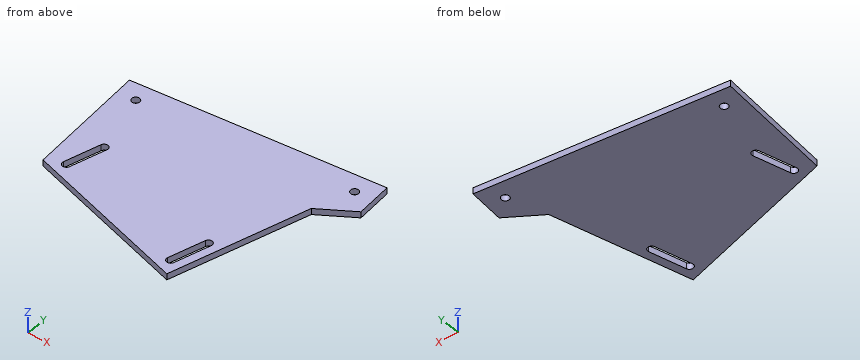
```python
from build123d import *

# Parameters (mm, degrees)
SKETCH2_R           = 4.1021
BOSS_EXTRUDE2_DEPTH = 6.35


with BuildPart() as part:
    # Sketch2 → Boss-Extrude2 (new body)
    with BuildSketch(Plane.XY):
        Polygon((416.876840794, 161.047876949), (163.843387479, 138.910318291), (174.883865248, 12.717079939), (347.922940958, -40.266575593), (385.763827966, 100.957537323), (420.197474593, 123.092858952), align=None)
        with Locations((184.481213377, 121.593126192)):
            Circle(SKETCH2_R, mode=Mode.SUBTRACT)
        with Locations((399.559648695, 140.410051051)):
            Circle(SKETCH2_R, mode=Mode.SUBTRACT)
        with BuildLine():
            Line((352.884248555, 11.469011076), (343.023242936, -25.332762905))
            ThreePointArc((343.023242936, -25.332762905), (337.999216999, -28.233385633), (335.098594272, -23.209359696))
            Line((335.098594272, -23.209359696), (344.959599891, 13.592414286))
            ThreePointArc((344.959599891, 13.592414286), (349.983625828, 16.493037013), (352.884248555, 11.469011076))
        make_face(mode=Mode.SUBTRACT)
        with BuildLine():
            ThreePointArc((199.237675668, 58.211701605), (204.261701605, 61.112324332), (207.162324332, 56.088298395))
            Line((207.162324332, 56.088298395), (197.301318714, 19.286524413))
            ThreePointArc((197.301318714, 19.286524413), (192.277292777, 16.385901686), (189.37667005, 21.409927623))
            Line((189.37667005, 21.409927623), (199.237675668, 58.211701605))
        make_face(mode=Mode.SUBTRACT)
    extrude(amount=BOSS_EXTRUDE2_DEPTH)


solid = part.part
```
Design review of the part built by this model. Coordinates are the model's own, in mm. Give positions to 0.01 mm unless a question says otherwise; leave off trailing zeros. Order: outer loops, then holes, each group sorted by start corner. A loop starts at its lowest first (then second) coordinate and runs counter-clockwise, first axis right, second up. Notation, with made-up numbers: (42.25, -4.75) - (66.25, -4.75) arc R21 ccw to (66.25, 18.25) - close; hole circle Ø4 at (43, -19). An arc over 180 degrees is marked (long way). Use a Markdown table: item, result. Add a question column.
(1) Add section B-B on z = 1. Give the boundary of the cut face in (x, y).
(2) Add section A-A on x = 203.2. Give the boundary of the cut face in (y, z).
(3) Wall thickness on probe 1 along X at (y, z) = (14.5, 5.25); probe 2 along X at (y, z) = (37, 4.25); probe 3 along Y at (x, z) = (182.5, 5.5): over which ranges is each line inside the solid? List them lowest first. Write a range as [from, to].
(4) Add section C-C on y = 149. Give the boundary of the cut face in (x, z), then the cut area to 3 significant figures.
(5) Clearance check with flat-ended pins moving along their axes: P1, Ø1, axis at x = 368.5, y = 59, coming from the -Z side; P2, Ø1, axis at x = 219, z = 3.5, coming from the -Y side; P3, Ø2, axis at x = 230, z = 3, coming from the +Y side. State where each tip first meets the part, or that it passes through.
(6) Add section D-D on x = 381.5. Give the boundary of the cut face in (y, z).
Report:
| question | item | result |
|---|---|---|
| 1 | outline | (163.84, 138.91) - (174.88, 12.72) - (347.92, -40.27) - (385.76, 100.96) - (420.2, 123.09) - (416.88, 161.05) - close; hole circle Ø8.2 at (184.48, 121.59); hole (189.38, 21.41) arc R4.1 ccw to (197.3, 19.29) - (207.16, 56.09) arc R4.1 ccw to (199.24, 58.21) - close; hole (335.1, -23.21) arc R4.1 ccw to (343.02, -25.33) - (352.88, 11.47) arc R4.1 ccw to (344.96, 13.59) - close; hole circle Ø8.2 at (399.56, 140.41) |
| 2 | outline | (4.05, 0) - (41.3, 0) - (41.3, 6.35) - (4.05, 6.35) - close; (61.25, 0) - (142.35, 0) - (142.35, 6.35) - (61.25, 6.35) - close |
| 3 | probe 1 | x = [174.73, 345.32], [352.52, 362.6] |
| 3 | probe 2 | x = [172.76, 193.55], [202.05, 368.63] |
| 3 | probe 3 | y = [10.39, 118], [125.19, 140.54] |
| 4 | outline | (279.17, 0) - (417.93, 0) - (417.93, 6.35) - (279.17, 6.35) - close |
| 4 | area | 881 mm² |
| 5 | P1 | stops at z = 0 |
| 5 | P2 | stops at y = -0.94 |
| 5 | P3 | stops at y = 144.79 |
| 6 | outline | (85.04, 0) - (157.95, 0) - (157.95, 6.35) - (85.04, 6.35) - close |
